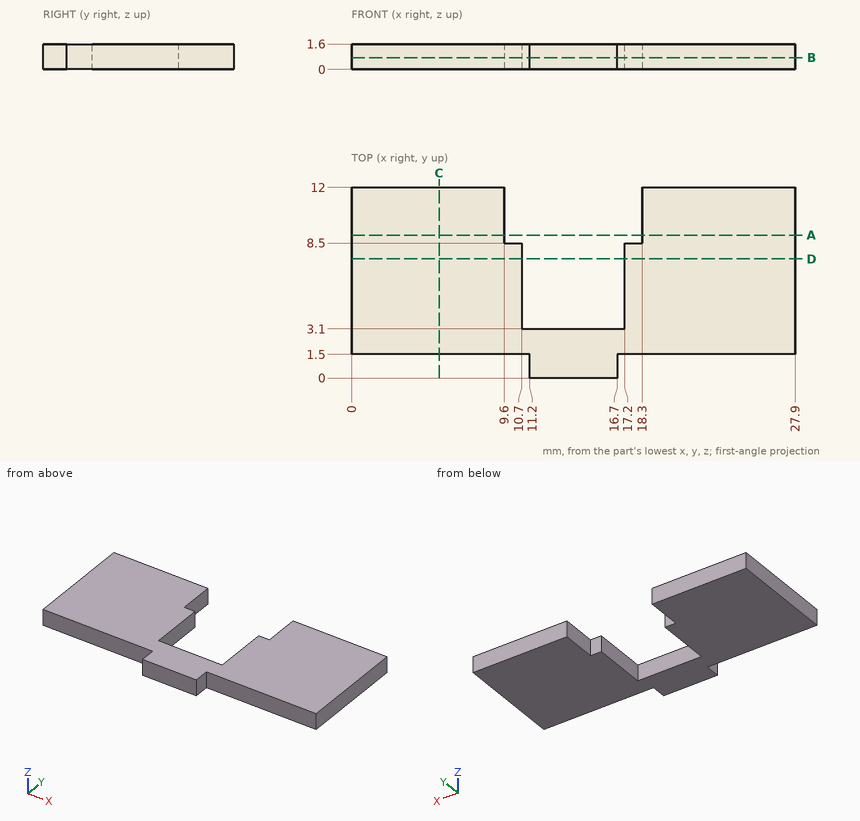
Here's the drawing with two shaded views (mm, measured from the low corner). I have some questions. Coordinates: 2 decimals unless noted, no trailing zeros. Write each loop counter-clockwise with the first axis right and the second up, starting at its lowest first coordinate (ties: lowest second). Pieces come first, ordered by that corner, then holes.
Item 1: I want a section at B-B on z = 0.75. Write out the boundary of the cut face in (x, y), and give its area (3 significant figures).
Item 2: Will these pins go through, and if not, where does the flat tip stop? pin 1 (0.5 mm diameter, centred on x = 10.5, z = 0.5, fed in from +Y); pin 2 (0.5 mm diameter, centred on x = 21, z = 1, fed in from -Y); pin 3 (0.5 mm diameter, centred on x = 14.5, z = 0.5, fed in from +Y).
Item 3: I want a section at C-C on x = 5.5. Write out the boundary of the cut face in (y, z), and give its area (3 significant figures).
Item 4: I want a section at D-D on y = 7.5. Write out the boundary of the cut face in (x, z).
Item 5: If I drill on line 1 (X direction, y = 7, z = 0.45); line 2 (X direction, y = 9.5, z = 0.2); line 3 (Y direction, x = 10.5, z = 0.8), over which ranges is the centre line in solid material (lowest first)?
Item 6: I want a section at A-A on y = 9. Write out the boundary of the cut face in (x, z).
Findings below:
1. outline: (0, 1.5) - (11.2, 1.5) - (11.2, 0) - (16.7, 0) - (16.7, 1.5) - (27.9, 1.5) - (27.9, 12) - (18.3, 12) - (18.3, 8.5) - (17.2, 8.5) - (17.2, 3.1) - (10.7, 3.1) - (10.7, 8.5) - (9.6, 8.5) - (9.6, 12) - (0, 12) - close
1. area: 236 mm2
2. pin 1: stops at y = 8.5
2. pin 2: stops at y = 1.5
2. pin 3: stops at y = 3.1
3. outline: (1.5, 0) - (12, 0) - (12, 1.6) - (1.5, 1.6) - close
3. area: 16.8 mm2
4. outline: (0, 0) - (10.7, 0) - (10.7, 1.6) - (0, 1.6) - close; (17.2, 0) - (27.9, 0) - (27.9, 1.6) - (17.2, 1.6) - close
5. line 1: x = 0 to 10.7, 17.2 to 27.9
5. line 2: x = 0 to 9.6, 18.3 to 27.9
5. line 3: y = 1.5 to 8.5
6. outline: (0, 0) - (9.6, 0) - (9.6, 1.6) - (0, 1.6) - close; (18.3, 0) - (27.9, 0) - (27.9, 1.6) - (18.3, 1.6) - close
